from build123d import *

# Parameters (mm, degrees)
RESSALTO_EXTRUS_O1_DEPTH                           = 1.5
ESBO_O2_R                                          = 17
CORTE_EXTRUS_O1_DEPTH                              = 1.5
FURO_ROSCADO_DE_M21_D                              = 1.6
CORTE_EXTRUS_O3_DEPTH                              = 1.5
ESCAREADO_PARA_PARAFUSO_COM_CABE_A_E_2_COUNT       = 2
ESCAREADO_PARA_PARAFUSO_COM_CABE_A_E_2_PITCH       = 7
ESCAREADO_PARA_PARAFUSO_COM_CABE_A_E_3_COUNT       = 2
ESCAREADO_PARA_PARAFUSO_COM_CABE_A_E_3_PITCH       = 42.234139035
ESCAREADO_PARA_PARAFUSO_COM_CABE_A_E_4_COUNT       = 2
ESCAREADO_PARA_PARAFUSO_COM_CABE_A_E_4_PITCH       = 41.65
ESCAREADO_PARA_PARAFUSO_COM_CABE_A_E_5_COUNT       = 2
ESCAREADO_PARA_PARAFUSO_COM_CABE_A_E_5_PITCH       = 83.568902959
ESCAREADO_PARA_PARAFUSO_COM_CABE_A_E_6_COUNT       = 2
ESCAREADO_PARA_PARAFUSO_COM_CABE_A_E_6_PITCH       = 81.286400606
ESCAREADO_PARA_PARAFUSO_COM_CABE_A_E_7_COUNT       = 2
ESCAREADO_PARA_PARAFUSO_COM_CABE_A_E_7_PITCH       = 47.258735882
ESCAREADO_PARA_PARAFUSO_COM_CABE_A_E_8_COUNT       = 2
ESCAREADO_PARA_PARAFUSO_COM_CABE_A_E_8_PITCH       = 43.094146922
ESCAREADO_PARA_PARAFUSO_COM_CABE_A_E_9_D           = 3.4
ESCAREADO_PARA_PARAFUSO_COM_CABE_A_E_9_DEPTH       = 7.25
ESCAREADO_PARA_PARAFUSO_COM_CABE_A_E_9_CSINK_D     = 6.3
ESCAREADO_PARA_PARAFUSO_COM_CABE_A_E_9_CSINK_ANGLE = 90
ESCAREADO_PARA_PARAFUSO_COM_CABE_A_E_9_TIP         = 1.021463052
CORTE_EXTRUS_O7_DEPTH                              = 122.865704775
CORTE_EXTRUS_O8_DEPTH                              = 114.698293533
FILETE1_R                                          = 2
BROCA_DE_ROSQUEAR_PARA_TARRAXA_DE_M31_D            = 2.5


with BuildPart() as part:
    # Esboço1 → Ressalto-extrusão1 (new body)
    with BuildSketch(Plane.XY):
        with BuildLine():
            Line((-17, 85.322916031), (-17, -85.322916031))
            ThreePointArc((-17, -85.322916031), (-87, 0), (-17, 85.322916031))
        make_face()
    extrude(amount=RESSALTO_EXTRUS_O1_DEPTH)

    # Esboço2 → Corte-extrusão1 (cut)
    with BuildSketch(Plane.XY.offset(1.5)):
        with Locations((-61, 0)):
            Circle(ESBO_O2_R)
    extrude(amount=-CORTE_EXTRUS_O1_DEPTH, mode=Mode.SUBTRACT)

    # Furo roscado de M21 (through all)
    with Locations(Plane(origin=(-71, 17.320508076, 1.5), x_dir=(1, 0, 0), z_dir=(0, 0, 1))):
        with Locations((0, 0), (30, -17.320508076), (0, -34.641016152)):
            Hole(FURO_ROSCADO_DE_M21_D / 2)

    # Esboço6 → Corte-extrusão3 (cut)
    with BuildSketch(Plane.XY.offset(1.5)):
        with BuildLine():
            Line((-30, -24.445048467), (-30, 24.445048467))
            ThreePointArc((-30, 24.445048467), (-29.879385242, 25.129088753), (-29.532088886, 25.730623686))
            Line((-29.532088886, 25.730623686), (-17, 40.665785639))
            Line((-17, 40.665785639), (-17, -40.665785639))
            Line((-17, -40.665785639), (-29.532088886, -25.730623686))
            ThreePointArc((-29.532088886, -25.730623686), (-29.879385242, -25.129088753), (-30, -24.445048467))
        make_face()
    extrude(amount=-CORTE_EXTRUS_O3_DEPTH, mode=Mode.SUBTRACT)

    # Esboço11 → Escareado para parafuso com cabe_a escar (revolve, cut)
    with BuildSketch(Plane(origin=(-60.558332829, -23.629367941, 1.5), x_dir=(0, -1, 0), z_dir=(1, 0, 0))):
        Polygon((0, 0), (0, 1.5), (1.7, 1.5), (1.7, 1.45), (3.15, 0), align=None)
    escareado_para_parafuso_com_cabe_a_escar = revolve(axis=Axis((-60.558332829, -23.629367941, 7.85), (0, 0, -1)), mode=Mode.SUBTRACT)

    # Escareado para parafuso com cabe_a e 2: Escareado para parafuso com cabe_a escar ×2
    with Locations(*[Vector(0.7660444431189771, 0.6427876096865406, 0) * (i * ESCAREADO_PARA_PARAFUSO_COM_CABE_A_E_2_PITCH) for i in range(1, ESCAREADO_PARA_PARAFUSO_COM_CABE_A_E_2_COUNT)]):
        add(escareado_para_parafuso_com_cabe_a_escar, mode=Mode.SUBTRACT)

    # Escareado para parafuso com cabe_a e 3: Escareado para parafuso com cabe_a escar ×2
    with Locations(*[Vector(0.7608635047324315, -0.6489119564057063, 0) * (i * ESCAREADO_PARA_PARAFUSO_COM_CABE_A_E_3_PITCH) for i in range(1, ESCAREADO_PARA_PARAFUSO_COM_CABE_A_E_3_COUNT)]):
        add(escareado_para_parafuso_com_cabe_a_escar, mode=Mode.SUBTRACT)

    # Escareado para parafuso com cabe_a e 4: Escareado para parafuso com cabe_a escar ×2
    with Locations(*[Vector(0.6427876096865411, -0.7660444431189766, 0) * (i * ESCAREADO_PARA_PARAFUSO_COM_CABE_A_E_4_PITCH) for i in range(1, ESCAREADO_PARA_PARAFUSO_COM_CABE_A_E_4_COUNT)]):
        add(escareado_para_parafuso_com_cabe_a_escar, mode=Mode.SUBTRACT)

    # Escareado para parafuso com cabe_a e 5: Escareado para parafuso com cabe_a escar ×2
    with Locations(*[Vector(0.3203596433075423, 0.9472959933093058, 0) * (i * ESCAREADO_PARA_PARAFUSO_COM_CABE_A_E_5_PITCH) for i in range(1, ESCAREADO_PARA_PARAFUSO_COM_CABE_A_E_5_COUNT)]):
        add(escareado_para_parafuso_com_cabe_a_escar, mode=Mode.SUBTRACT)

    # Escareado para parafuso com cabe_a e 6: Escareado para parafuso com cabe_a escar ×2
    with Locations(*[Vector(0.3953233850400935, 0.9185420084244608, 0) * (i * ESCAREADO_PARA_PARAFUSO_COM_CABE_A_E_6_PITCH) for i in range(1, ESCAREADO_PARA_PARAFUSO_COM_CABE_A_E_6_COUNT)]):
        add(escareado_para_parafuso_com_cabe_a_escar, mode=Mode.SUBTRACT)

    # Escareado para parafuso com cabe_a e 7: Escareado para parafuso com cabe_a escar ×2
    with Locations(*[(0, i * ESCAREADO_PARA_PARAFUSO_COM_CABE_A_E_7_PITCH, 0) for i in range(1, ESCAREADO_PARA_PARAFUSO_COM_CABE_A_E_7_COUNT)]):
        add(escareado_para_parafuso_com_cabe_a_escar, mode=Mode.SUBTRACT)

    # Escareado para parafuso com cabe_a e 8: Escareado para parafuso com cabe_a escar ×2
    with Locations(*[Vector(0.12443246902051158, 0.9922280789483129, 0) * (i * ESCAREADO_PARA_PARAFUSO_COM_CABE_A_E_8_PITCH) for i in range(1, ESCAREADO_PARA_PARAFUSO_COM_CABE_A_E_8_COUNT)]):
        add(escareado_para_parafuso_com_cabe_a_escar, mode=Mode.SUBTRACT)

    # Escareado para parafuso com cabe_a e 9
    with Locations(Plane(origin=(-48.209070726, -57.453333234, 0), x_dir=(-1, 0, 0), z_dir=(0, 0, -1))):
        with Locations((0, 0), (16.742834558, 19.953333234), (16.742834558, 94.953333234), (4.823937863, 110.486341823)):
            CounterSinkHole(ESCAREADO_PARA_PARAFUSO_COM_CABE_A_E_9_D / 2, ESCAREADO_PARA_PARAFUSO_COM_CABE_A_E_9_CSINK_D / 2, depth=ESCAREADO_PARA_PARAFUSO_COM_CABE_A_E_9_DEPTH, counter_sink_angle=ESCAREADO_PARA_PARAFUSO_COM_CABE_A_E_9_CSINK_ANGLE)
            with Locations((0, 0, -(ESCAREADO_PARA_PARAFUSO_COM_CABE_A_E_9_DEPTH + ESCAREADO_PARA_PARAFUSO_COM_CABE_A_E_9_TIP / 2))):  # 118° drill point
                Cone(0, ESCAREADO_PARA_PARAFUSO_COM_CABE_A_E_9_D / 2, ESCAREADO_PARA_PARAFUSO_COM_CABE_A_E_9_TIP, mode=Mode.SUBTRACT)

    # Esboço19 → Corte-extrusão7 (cut, through all)
    with BuildSketch(Plane(origin=(0, 0, 0), x_dir=(-1, 0, 0), z_dir=(0, 0, -1))):
        Polygon((31.215078447, 58.599296769), (17, 46.671429688), (17, 85.322916031), (63.063047709, 85.322916031), align=None)
        Polygon((30.572290837, -59.365341213), (17, -47.976836977), (17, -85.322916031), (61.507323882, -85.322916031), align=None)
    extrude(amount=-CORTE_EXTRUS_O7_DEPTH, mode=Mode.SUBTRACT)

    # Esboço20 → Corte-extrusão8 (cut, through all)
    with BuildSketch(Plane(origin=(0, 0, 0), x_dir=(-1, 0, 0), z_dir=(0, 0, -1))):
        with BuildLine():
            Line((47.91785698, 72.614592076), (45.51622644, 70.599384776))
            ThreePointArc((45.51622644, 70.599384776), (83.998363098, -0.524401402), (44.631209662, -71.162174813))
            Line((44.631209662, -71.162174813), (47.04198176, -73.185052792))
            ThreePointArc((47.04198176, -73.185052792), (86.998430183, -0.522633435), (47.91785698, 72.614592076))
        make_face()
    extrude(amount=-CORTE_EXTRUS_O8_DEPTH, mode=Mode.SUBTRACT)

    # Filete1
    filete1_edges = [part.edges().sort_by_distance(p)[0] for p in [
        (-17, 46.671429688, 0.75),
        (-17, -47.976836977, 0.75),
        (-45.51622644, 70.599384776, 0.75),
        (-44.631209662, -71.162174813, 0.75),
        (-17, 40.665785639, 0.75),
        (-17, -40.665785639, 0.75),
    ]]
    fillet(filete1_edges, radius=FILETE1_R)

    # Broca de rosquear para tarraxa de M31 (through all)
    with Locations(Plane(origin=(-30, -44, 1.5), x_dir=(1, 0, 0), z_dir=(0, 0, 1))):
        with Locations((0, 0), (0, 8), (0, 88), (0, 80)):
            Hole(BROCA_DE_ROSQUEAR_PARA_TARRAXA_DE_M31_D / 2)


solid = part.part
The model under review builds one solid part; all positions refer to its coordinate system, in mm. A direction names the side the tool comes from. Round coordinates to 2 decimals unless told otherwise and drop trailing zeros. Order: outer loops, then holes, each group sorted by start corner. A loop starts at its lowest first (then second) coordinate and runs counter-clockwise, first axis right, second up. Notation, with made-up numbers: (25.25, -30.5) -> (45.25, -30.5) arc R22 ccw to (45.25, 4.5) -> close; hole circle Ø2 at (12, 14). An arc over 180 degrees is marked (long way). Write item = value, one per line. Start each with the question number.
Item 1: Consider section C-C on z = 0.55. Count the separate pieces of the cut face and the enclosed holes in it, plus the area to 3 significant figures.
Item 2: Mouldability with a two-part tool opening along X and no side actions: class faces 1 (the face through (-31.155, -36.479, 0.739)), 2 (the face through (-43, 1, 1.5)), 3 (the face through (-83.998, 0.626, 0.74)) as released by +X, released by -X, zero draft, split by the parting line, or undercut.
Item 3: Consider section B-B on y = 12.5. Write out the cut boundary in (x, z), plus the area to 3 significant figures.
Item 4: Consider section A-A on y = 44. Write out the cut boundary in (x, z).
Item 5: For line 1 along Y through (x, z) = (-64.5, 0.5); line 2 along Y through (x, z) = (-70.5, 0.8) (3 decimals); line 3 along Y through (x, z) = (-31, 0.65), list the stretches that pass through material, from the lowest coordinate up.
Item 6: Consider section D-D on y = -30. Write out the cut boundary in (x, z).
Item 7: Clearance check with flat-ended pins moving along their axes: pin 1 Ø4.5 at (x, y) = (-48.21, -57.45) entering from -Z; pin 2 Ø4.5 at (x, y) = (-60.56, -23.63) entering from +Z; pin 3 Ø5.5 at (x, y) = (-53.03, 53.03) entering from -Z. State where each tip first meets the part, or that it passes through.
Item 8: For faces 4 (the face through (-23.6, 32.8, 0.8)), 5 (the face through (-29.84, -42.76, 0.74)), list the 3-axis set-ups (+Z, -Z, +X, -X, +Y, -Y) from which the entire face can be reached by the end or side of a thin tool; tool diameter is ignored.
Conclusion:
q1.separate_pieces = 1
q1.enclosed_holes = 20
q1.area = 5,210 mm2
q2.face_1 = undercut
q2.face_2 = zero draft
q2.face_3 = released by -X
q3.outline = (-83.06, 0) -> (-72.52, 0) -> (-72.52, 1.5) -> (-83.06, 1.5) -> close; (-49.48, 0) -> (-30, 0) -> (-30, 1.5) -> (-49.48, 1.5) -> close
q3.area = 45.0 mm2
q4.outline = (-71.55, 0) -> (-31.25, 0) -> (-31.25, 1.5) -> (-71.55, 1.5) -> close; (-28.75, 0) -> (-17, 0) -> (-17, 1.5) -> (-28.75, 1.5) -> close
q5.line_1 = -53.81 to -40.11, -34.89 to -16.64, 16.64 to 34.89, 40.11 to 53.81
q5.line_2 = -45.67 to -17.945, -16.696 to -14.098, 14.098 to 16.696, 17.945 to 45.67
q5.line_3 = -59.72 to -44.75, -43.25 to -36.75, -35.25 to 35.25, 36.75 to 43.25, 44.75 to 58.42
q6.outline = (-78.46, 0) -> (-25.95, 0) -> (-25.95, 1.5) -> (-78.46, 1.5) -> close
q7.pin_1 = 0.9
q7.pin_2 = 0.6
q7.pin_3 = 0.4
q8.face_4 = +Z, -Z, +X
q8.face_5 = +Z, -Z
